Geometry: final body of the model. Coordinates: model frame, mm. Face numbers are marked on the shaded views. A direction names the side the tool comes from. Give positions to 0.01 mm unless a question says otherwise; leave off trailing zeros. Order: outer loops, then holes, each group sorted by start corner. A loop starts at its lowest first (then second) coordinate and runs counter-clockwise, first axis right, second up. Notation, with made-up numbers: M 50,-30.5 L 95,-30.5 A25 ccw 95,-18.5 Z; hole C 70.5,81 d7. An arc over 180 degrees is marked long. Write item = value, one per line. Start each with the question number.
Autodesk Inventor part; units mm, degrees
ref_plane "YZ Plane" through (0, 0, 0) normal (1, 0, 0) x (0, 1, 0)
ref_plane "XZ Plane" through (0, 0, 0) normal (0, 1, 0) x (-1, 0, 0)
ref_plane "XY Plane" through (0, 0, 0) normal (0, 0, 1) x (1, 0, 0)
sketch "Sketch1" plane through (0, 0, 0) normal (0, 0, 1) x (1, 0, 0)
  circle A0 centre (0, 0) radius 45.75
  circle A1 centre (0, 0) radius 46.75
  line L0 (45.75, -0.0157) -> (46.75, -0.0157) construction
  line L1 (42.7149, 19) -> (121.75, 19)
  line L2 (121.75, 19) -> (121.75, -19)
  line L3 (121.75, -19) -> (42.7149, -19)
  line L4 (41.768, 21) -> (123.75, 21)
  line L5 (123.75, 21) -> (123.75, -21)
  line L6 (123.75, -21) -> (41.768, -21)
  line L7 (82.759, 21) -> (82.759, 19) construction
  line L8 (121.75, 0) -> (123.75, 0) construction
  line L9 (98.0367, -19) -> (98.0367, -21) construction
  line L10 (0, 0) -> (121.75, 0) construction
  line L11 (41.768, 21) -> (40.6456, 21)
  line L12 (41.768, -21) -> (40.6456, -21)
  dimension "d0" = 91.5
  dimension "d2" = 1
  dimension "d3" = 75
  dimension "d4" = 38
  dimension "d5" = 2
extrude "Extrusion1" add sketch "Sketch1" along normal blind 20 contours A0 L11 A1 L12 | A0 L12 A1 L11
extrude "Extrusion2" add sketch "Sketch1" along normal blind 2 contours L4 L5 L6 A1 L3 L2 L1 | L1 L2 L3 A1
extrude "Extrusion9" add sketch "Sketch1" along normal blind 40 contours A0 L11 A1 L12 | L4 L5 L6 A1 L3 L2 L1 picked at (42.2726, -18.1004)
sketch "Sketch8" plane through (123.75, -21, 0) normal (1, 0, 0) x (0, 0, -1)
  line L0 (0, 0) -> (0, 42)
  line L1 (0, 42) -> (-40, 42)
  line L2 (-40, 0) -> (-40, 42)
  line L3 (0, 0) -> (-40, 0)
  circle A0 centre (-12, 21) radius 4.05
  line L4 (-12, 21) -> (-12, 42) construction
  line L5 (-12, 21) -> (-12, 0) construction
  circle A1 centre (-28, 30) radius 3.25
  circle A2 centre (-28, 12) radius 3.25
  line L6 (-28, 30) -> (-28, 12) construction
  line L7 (-40, 21) -> (-28, 21) construction
  point P0 (0, 21)
  dimension "d40" = 8.1
  dimension "d42" = 12
  dimension "d43" = 6.5
  dimension "d44" = 12
  dimension "d61" = 18
extrude "Extrusion10" cut sketch "Sketch8" against normal up to surface (2 mm away) contours A0 | A1 | A2
sketch "Sketch9" plane through (0, 0, 2) normal (0, 0, 1) x (1, 0, 0)
  arc A0 (42.7149, -19) -> (42.7149, 19) centre (0, 0) ccw
  line L0 (42.7149, -19) -> (121.75, -19)
  line L1 (46.75, 0) -> (81.75, 0) construction
  line L2 (81.75, 19) -> (89.75, 19)
  line L3 (89.75, 19) -> (89.75, 9.25)
  line L4 (89.75, 9.25) -> (81.75, 9.25)
  line L5 (81.75, 9.25) -> (81.75, 19)
  line L6 (81.75, -19) -> (89.75, -19)
  line L7 (89.75, -19) -> (89.75, -9.25)
  line L8 (89.75, -9.25) -> (81.75, -9.25)
  line L9 (81.75, -9.25) -> (81.75, -19)
  line L10 (81.75, 19) -> (81.75, -19) construction
  line L11 (42.7149, 19) -> (121.75, 19)
  line L12 (89.75, -19) -> (81.75, -19)
  dimension "d49" = 35
  dimension "d52" = 18.5
  dimension "d53" = 8
extrude "Extrusion11" add sketch "Sketch9" along normal blind 15
sketch "Sketch10" plane through (0, 0, 17) normal (0, 0, 1) x (1, 0, 0)
  line L0 (81.75, 19) -> (89.75, 19)
  line L1 (81.75, 19) -> (81.75, 9.25)
  line L2 (81.75, 9.25) -> (89.75, 9.25)
  line L3 (89.75, 9.25) -> (89.75, 19)
  line L4 (89.75, -19) -> (89.75, -9.25)
  line L5 (89.75, -9.25) -> (81.75, -9.25)
  line L6 (81.75, -9.25) -> (81.75, -19)
  line L7 (89.75, -19) -> (81.75, -19)
  circle A0 centre (85.75, -14.125) radius 2.1
  circle A1 centre (85.75, 14.125) radius 2.1
  line L8 (89.75, 19) -> (81.75, 9.25) construction
  line L9 (89.75, -9.25) -> (81.75, -19) construction
  point P0 (0, 0)
  dimension "d58" = 4.2
extrude "Extrusion12" cut sketch "Sketch10" against normal blind 5 contours A0 | A1
properties part number "Pump enclosure MM0312"
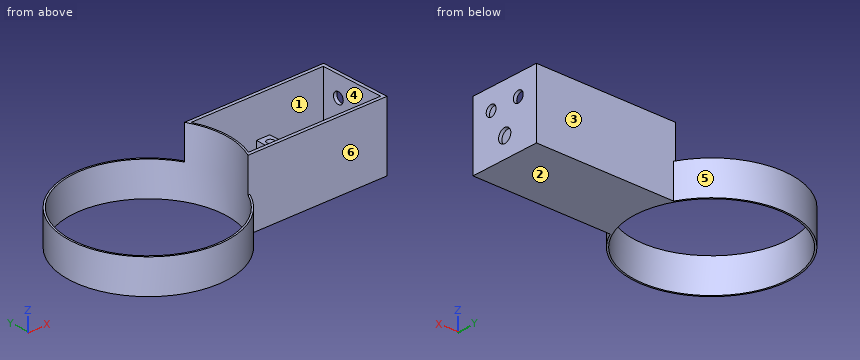
1) Access query for the marked faces 1 and 2. Directions: +Z, -Z, +X, -X, +Y, -Y. A direction counts if a zero-diameter tool reaches every point of the face in a straight line with its end or side. Return the directions, or none.
2) Cut plane C-C (x = 85.75). Return loops of the section in (y, z) (3 decimals).
3) Ray query, L1, parallel to Y at x = 85.75, z = 15.25 (3 decimals); L2, parallel to Y at x = 122.35, z = 28; L3, parallel to X at y = 7, z = 17. Return the intervals inside material, ascending.
4) Pin query (flat end, axial travel): pin 1 Ø11.5 at (y, z) = (-2, 24) entering from -X; pin 2 Ø11.5 at (x, z) = (92.5, 23.5) entering from -Y; pin 3 Ø4 at (x, y) = (85.75, 14.125) entering from +Z. Return the tip coordinate at first contact, or that it passes through.
5) Cut plane D-D (z = 37). Return loops of the section in (x, y).
6) Cut plane A-A (z = 27). Return loops of the section in (x, y), plus the area to 3 significant figures.
7) Draft query along Y for the marked faces 3, 4, 5 and 6. Return one class per face: pulls with the +Y half, pulls with the -Y half, needs draft (parallel to the pull), parting line crosses it, or undercut.
8) Cut plane B-B (x = -5.5). Return loops of the section in (y, z), plus the area to 3 significant figures.
Reply:
q1.face_1 = +Z
q1.face_2 = -Z, +X, -X, +Y, -Y
q2.outline = M -21,0 L 21,0 L 21,40 L 19,40 L 19,17 L 16.225,17 L 16.225,12 L 12.025,12 L 12.025,17 L 9.25,17 L 9.25,2 L -9.25,2 L -9.25,17 L -12.025,17 L -12.025,12 L -16.225,12 L -16.225,17 L -19,17 L -19,40 L -21,40 Z
q3.L1 = -21 to -16.225, -12.025 to -9.25, 9.25 to 12.025, 16.225 to 21
q3.L2 = -21 to -12.25, -5.75 to 5.75, 12.25 to 21
q3.L3 = -46.22 to -45.21, 45.21 to 46.22, 121.75 to 123.75
q4.pin_1 = -46.75
q4.pin_2 = -21
q4.pin_3 = 12
q5.outline = M 40.65,-21 L 123.75,-21 L 123.75,21 L 40.65,21 A45.75 cw Z; hole M 42.71,-19 L 121.75,-19 L 121.75,19 L 42.71,19 A46.75 cw Z
q6.outline = M 40.65,-21 L 123.75,-21 L 123.75,-12.09 L 121.75,-12.09 L 121.75,-19 L 42.71,-19 A46.75 ccw 42.71,19 L 121.75,19 L 121.75,12.09 L 123.75,12.09 L 123.75,21 L 40.65,21 A45.75 cw Z; M 121.75,-5.91 L 123.75,-5.91 L 123.75,5.91 L 121.75,5.91 Z
q6.area = 421 mm²
q7.face_3 = pulls with the +Y half
q7.face_4 = undercut
q7.face_5 = parting line crosses it
q7.face_6 = pulls with the -Y half
q8.outline = M -46.43,0 L -45.42,0 L -45.42,20 L -46.43,20 Z; M 45.42,0 L 46.43,0 L 46.43,20 L 45.42,20 Z
q8.area = 40.3 mm²
